from build123d import *

# Parameters (mm, degrees)
SKETCH1_W           = 63.5
SKETCH1_H           = 76.2
SKETCH1_R           = 3.175
SKETCH1_W_2         = 12.7
BOSS_EXTRUDE1_DEPTH = 6.35
SKETCH2_W           = 12.7
SKETCH2_H           = 76.2
CUT_EXTRUDE1_DEPTH  = 2.54
CUT_EXTRUDE2_DEPTH  = 108.95


with BuildPart() as part:
    # Sketch1 → Boss-Extrude1 (new body)
    # profile 1 of 2: a face of its own
    with BuildSketch(Plane(origin=(0, 0, 0), x_dir=(1, 0, 0), z_dir=(0, 1, 0))):
        with Locations((31.75, 38.1)):
            Rectangle(SKETCH1_W, SKETCH1_H)
        with Locations(Location((19.177, 13.335, 0), (0, 0, 270))):
            Circle(SKETCH1_R, mode=Mode.SUBTRACT)
        with Locations(Location((19.177, 62.865, 0), (0, 0, 90))):
            Circle(SKETCH1_R, mode=Mode.SUBTRACT)
    # profile 2 of 2: a face of its own
    with BuildSketch(Plane(origin=(0, 0, 0), x_dir=(1, 0, 0), z_dir=(0, 1, 0))):
        with Locations((69.85, 38.1)):
            Rectangle(SKETCH1_W_2, SKETCH1_H)
    extrude(amount=BOSS_EXTRUDE1_DEPTH)

    # Sketch2 → Cut-Extrude1 (cut)
    with BuildSketch(Plane(origin=(0, 6.35, 0), x_dir=(1, 0, 0), z_dir=(0, 1, 0))):
        with Locations((69.85, 38.1)):
            Rectangle(SKETCH2_W, SKETCH2_H)
    extrude(amount=-CUT_EXTRUDE1_DEPTH, mode=Mode.SUBTRACT)

    # Sketch3 → Cut-Extrude2 (cut, through all)
    with BuildSketch(Plane(origin=(0, 6.35, 0), x_dir=(1, 0, 0), z_dir=(0, 1, 0))):
        with BuildLine():
            Line((0, 44.45), (12.7, 44.45))
            ThreePointArc((12.7, 44.45), (15.875, 41.275), (12.7, 38.1))
            Line((12.7, 38.1), (0, 38.1))
            Line((0, 38.1), (0, 44.45))
        make_face()
    extrude(amount=-CUT_EXTRUDE2_DEPTH, mode=Mode.SUBTRACT)


solid = part.part
Part model, mm, in its own coordinate system. A direction names the side the tool comes from. Round coordinates to 2 decimals unless told otherwise and drop trailing zeros. Write each loop counter-clockwise with the first axis right and the second up, starting at its lowest first coordinate (ties: lowest second). Pieces come first, ordered by that corner, then holes. Notation, with made-up numbers: M 22,84.25 L 56,84.25 A20 cw 56,96.25 Z; hole C 12.5,25 d4. An arc over 180 degrees is marked long. Return JSON: item names as keys, results as strings. Group by question number.
(1) Pin check, flat tips, straight feed: pin 1 Ø1.5 at (x, y) = (66, 4) entering from -Z; pin 2 Ø2 at (y, z) = (5.5, -28.5) entering from +X; pin 3 Ø10 at (x, z) = (70, -31) entering from +Y; pin 4 Ø5.5 at (x, z) = (19.177, -62.865) entering from -Y. Stop position of each tip, or through.
(2) Drill centre lines: probe 1 along Z at (x, y) = (10, 2.75); probe 2 along Z at (x, y) = (17, 5.75); probe 3 along Y at (x, z) = (66, -68). Where is each one in solid material? Low to high.
(3) Saw through at D-D on z = -23.5. Write the cut outline in (x, y), then the cut area to 3 significant figures.
(4) Two-plate mould, pull along Z, no slides. Class faces 4 (the face through (38, 3, -76.2)), 5 (the face through (70, 3.81, -39)), 6 (the face through (17.031, 3.131, -60.525)), 7 (the face through (15.874, 3.219, -41.345)): +Z half, -Z half, draft (parallel to the pull), parting line (faces both ways), or undercut.
(5) Which spindle directions (+Z, -Z, +X, -X, +Y, -Y) get a long thin tool onto all of the face, cutting with end or side? Do faces 1 (the face through (0, 3, -19)), 2 (the face through (6, 3, -38.1)), 3 (the face through (63.5, 5, -38)). Say none if no direction does.
(6) Saw through at C-C on y = 2.25. Write the cut outline in (x, z) (3 decimals), then the cut area to 3 significant figures.
(7) Saw through at B-B on x = 17. Write the cut outline in (y, z), then the cut area to 3 significant figures.
(8) Saw through at A-A on x = 8. Write the cut outline in (y, z).
Returned:
{
 "1": {"pin 1": "z = -76.2", "pin 2": "x = 63.5", "pin 3": "y = 3.81", "pin 4": "through"},
 "2": {"probe 1": "-76.2 to -44.45, -38.1 to 0", "probe 2": "-76.2 to -65.18, -60.55 to -15.65, -11.02 to 0", "probe 3": "0 to 3.81"},
 "3": {"outline": "M 0,0 L 76.2,0 L 76.2,3.81 L 63.5,3.81 L 63.5,6.35 L 0,6.35 Z", "area": "452 mm²"},
 "4": {"face 4": "-Z half", "face 5": "draft", "face 6": "undercut", "face 7": "undercut"},
 "5": {"face 1": "+Z, -Z, -X, +Y, -Y", "face 2": "-X, +Y, -Y", "face 3": "+Z, -Z, +X, +Y"},
 "6": {"outline": "M 0,-76.2 L 76.2,-76.2 L 76.2,0 L 0,0 L 0,-38.1 L 12.7,-38.1 A3.175 cw 12.7,-44.45 L 0,-44.45 Z; hole C 19.177,-62.865 d6.35; hole C 19.177,-13.335 d6.35", "area": "5,650 mm²"},
 "7": {"outline": "M 0,-76.2 L 6.35,-76.2 L 6.35,-65.18 L 0,-65.18 Z; M 0,-60.55 L 6.35,-60.55 L 6.35,-15.65 L 0,-15.65 Z; M 0,-11.02 L 6.35,-11.02 L 6.35,0 L 0,0 Z", "area": "425 mm²"},
 "8": {"outline": "M 0,-76.2 L 6.35,-76.2 L 6.35,-44.45 L 0,-44.45 Z; M 0,-38.1 L 6.35,-38.1 L 6.35,0 L 0,0 Z"}
}
